Check sheet for the modelled part. Datum: model origin and axes. Units: mm. Face numbers are marked on the shaded views. Round coordinates to 2 decimals unless told otherwise and drop trailing zeros. Write each loop counter-clockwise with the first axis right and the second up, starting at its lowest first coordinate (ties: lowest second). Pieces come first, ordered by that corner, then holes.
Item 1: Section check A-A, the plane y = 21. Record the cut outline in (x, z), plus the area to 3 significant figures.
Item 2: Section check C-C, the plane x = 66.5. Record the cut outline in (y, z), plus the area to 3 significant figures.
Item 3: Release check for a two-part mould opening along Y. For the marked faces 1 and 2 record: pulls with the +Y half, pulls with the -Y half, needs draft (parallel to the pull), parting line crosses it, or undercut.
Item 4: Depth check by flat-ended pin: pin 1 (18.5 mm diameter, centred on x = -25, y = 21, fed in from +Z); pin 2 (1.5 mm diameter, centred on x = 13, z = 5, fed in from +Y); pin 3 (1.5 mm diameter, centred on x = 11, z = 4, fed in from -Y). Enter the tip coordinate at first touch or a pass-through.
Item 5: Section check B-B, the plane z = 1.25. State how many separate pieces and enclosed holes the cut face has, plus the area to 3 significant figures.
Item 6: Material ranges on line 1 along Y through (x, z) = (2.5, 1.5); line 2 along X through (y, z) = (-19.5, 1.65); line 3 along Y through (x, z) = (-50, 2.1), recorded low to high.
Item 7: Section check D-D, the plane y = 63.5. Record the cut outline in (x, z), plus the area to 3 significant figures.
from build123d import *

# Parameters (mm, degrees)
SKETCH_W        = 150
SKETCH_H        = 145
PAD_DEPTH       = 3
SKETCH001_R     = 2
POCKET_DEPTH    = 5
SKETCH002_R     = 1.5
POCKET001_DEPTH = 3.001
SKETCH003_R     = 1.6
POCKET002_DEPTH = 3.001
SKETCH004_W     = 33
SKETCH004_H     = 26
PAD001_DEPTH    = 3
SKETCH005_W     = 27
SKETCH005_H     = 20
POCKET003_DEPTH = 3
SKETCH006_R     = 8
SKETCH006_R_2   = 15
SKETCH006_W     = 22
SKETCH006_H     = 36
SKETCH006_W_2   = 17.5
SKETCH006_H_2   = 18.5
POCKET004_DEPTH = 3.001


with BuildPart() as part:
    # Sketch → Pad (new body)
    with BuildSketch(Plane.XY):
        Rectangle(SKETCH_W, SKETCH_H)
    extrude(amount=PAD_DEPTH)

    # Sketch001 (on Face6 of Pad) → Pocket (cut)
    with BuildSketch(Plane.XY.offset(3)):
        with Locations((-50, -66.5)):
            Circle(SKETCH001_R)
        with Locations((50, -66.5)):
            Circle(SKETCH001_R)
        with Locations((-66.5, 63.5)):
            Circle(SKETCH001_R)
        with Locations((66.5, 63.5)):
            Circle(SKETCH001_R)
    extrude(amount=-POCKET_DEPTH, mode=Mode.SUBTRACT)

    # Sketch002 (on Face5 of Pocket) → Pocket001 (cut, through all)
    with BuildSketch(Plane.XY.offset(3)):
        with Locations((-40, 52.5)):
            Circle(SKETCH002_R)
        with Locations((18, 52.5)):
            Circle(SKETCH002_R)
        with Locations((-40, 3.5)):
            Circle(SKETCH002_R)
        with Locations((18, 3.5)):
            Circle(SKETCH002_R)
    extrude(amount=-POCKET001_DEPTH, mode=Mode.SUBTRACT)

    # Sketch003 (on Face5 of Pocket001) → Pocket002 (cut, through all)
    with BuildSketch(Plane.XY.offset(3)):
        with Locations((-50, -11.5)):
            Circle(SKETCH003_R)
        with Locations((-12, -11.5)):
            Circle(SKETCH003_R)
        with Locations((-50, -49.5)):
            Circle(SKETCH003_R)
        with Locations((-12, -49.5)):
            Circle(SKETCH003_R)
    extrude(amount=-POCKET002_DEPTH, mode=Mode.SUBTRACT)

    # Sketch004 (on Face5 of Pocket002) → Pad001 (join)
    with BuildSketch(Plane.XY.offset(3)):
        with Locations((13.5, -21.5)):
            Rectangle(SKETCH004_W, SKETCH004_H)
    extrude(amount=PAD001_DEPTH)

    # Sketch005 (on Face23 of Pad001) → Pocket003 (cut)
    with BuildSketch(Plane.XY.offset(6)):
        with Locations((13.5, -21.5)):
            Rectangle(SKETCH005_W, SKETCH005_H)
    extrude(amount=-POCKET003_DEPTH, mode=Mode.SUBTRACT)

    # Sketch006 (on Face5 of Pocket003) → Pocket004 (cut, through all)
    with BuildSketch(Plane.XY.offset(3)):
        with Locations((-25, 41)):
            Circle(SKETCH006_R)
        with Locations((2.5, 41)):
            Circle(SKETCH006_R)
        with Locations((-25, 21)):
            Circle(SKETCH006_R)
        with Locations((2.5, 21)):
            Circle(SKETCH006_R)
        with Locations((-30, -30)):
            Circle(SKETCH006_R_2)
        with Locations((17, -48)):
            Circle(SKETCH006_R)
        with Locations((45, -48)):
            Circle(SKETCH006_R)
        with Locations((-53, 41)):
            Circle(SKETCH006_R)
        with Locations((-53, 21)):
            Circle(SKETCH006_R)
        with Locations((39, 28)):
            Rectangle(SKETCH006_W, SKETCH006_H)
        with Locations((48.75, -22.25)):
            Rectangle(SKETCH006_W_2, SKETCH006_H_2)
    extrude(amount=-POCKET004_DEPTH, mode=Mode.SUBTRACT)


solid = part.part
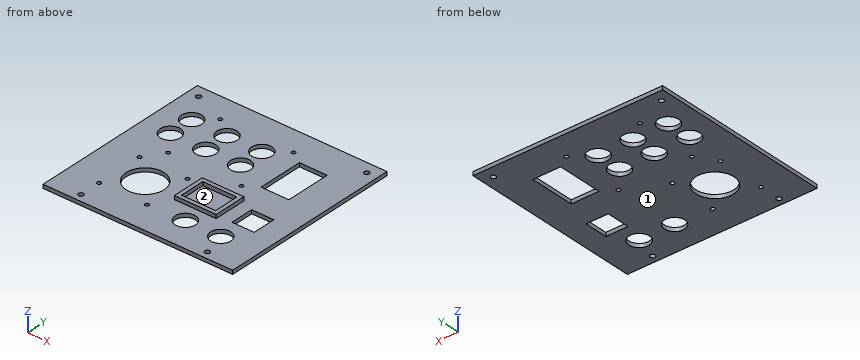
Values found:
1. outline: (-75, 0) - (-61, 0) - (-61, 3) - (-75, 3) - close; (-45, 0) - (-33, 0) - (-33, 3) - (-45, 3) - close; (-17, 0) - (-5.5, 0) - (-5.5, 3) - (-17, 3) - close; (10.5, 0) - (28, 0) - (28, 3) - (10.5, 3) - close; (50, 0) - (75, 0) - (75, 3) - (50, 3) - close
1. area: 240 mm2
2. outline: (-72.5, 0) - (61.5, 0) - (61.5, 3) - (-72.5, 3) - close; (65.5, 0) - (72.5, 0) - (72.5, 3) - (65.5, 3) - close
2. area: 423 mm2
3. face 1: needs draft
3. face 2: undercut
4. pin 1: stops at z = 3
4. pin 2: stops at y = -8.5
4. pin 3: stops at y = -34.5
5. separate pieces: 1
5. enclosed holes: 23
5. area: 18,200 mm2
6. line 1: y = -72.5 to 13, 29 to 33, 49 to 72.5
6. line 2: x = -75 to -40.71, -19.29 to 40, 57.5 to 75
6. line 3: y = -72.5 to -68.5, -64.5 to -51.1, -47.9 to -13.1, -9.9 to 13.58, 28.42 to 33.58, 48.42 to 72.5
7. outline: (-75, 0) - (-68.5, 0) - (-68.5, 3) - (-75, 3) - close; (-64.5, 0) - (64.5, 0) - (64.5, 3) - (-64.5, 3) - close; (68.5, 0) - (75, 0) - (75, 3) - (68.5, 3) - close
7. area: 426 mm2
